Autodesk Inventor part; units mm, degrees
ref_plane "YZ Plane" through (0, 0, 0) normal (1, 0, 0) x (0, 1, 0)
ref_plane "XZ Plane" through (0, 0, 0) normal (0, 1, 0) x (-1, 0, 0)
ref_plane "XY Plane" through (0, 0, 0) normal (0, 0, 1) x (1, 0, 0)
sketch "Sketch1" plane through (0, 0, 0) normal (0, 1, 0) x (-1, 0, 0)
  line L0 (0, 0) -> (-60, 0)
  line L1 (-60, 0) -> (-60, -26)
  line L2 (-60, -26) -> (0, -26)
  line L3 (0, -26) -> (0, 0)
  line L4 (-54, -3.5) -> (-6, -3.5)
  line L5 (-6, -3.5) -> (-6, -22.5)
  line L6 (-6, -22.5) -> (-54, -22.5)
  line L7 (-54, -22.5) -> (-54, -3.5)
  line L8 (-54, -3.5) -> (-6, -22.5) construction
  line L9 (-6, -3.5) -> (-54, -22.5) construction
  point P0 (-30, -13)
  dimension "d0" = 60
  dimension "d2" = 48
  dimension "d3" = 6
  dimension "d4" = 6
  dimension "d36" = 19
  dimension "d37" = 3.5
  dimension "d38" = 3.5
  dimension "d39" = 26
extrude "Extrusion1" add sketch "Sketch1" along normal blind 2 contours L3 L2 L1 L0 | L4 L5 L6 L7
extrude "Extrusion2" add sketch "Sketch1" along normal blind 19
sketch "Sketch2" plane through (0, 2, 0) normal (0, 1, 0) x (1, 0, 0)
  line L0 (6, 3.5) -> (54, 3.5)
  line L1 (54, 22.5) -> (6, 22.5)
  line L2 (54, 3.5) -> (48, 3.5)
  line L3 (48, 3.5) -> (48, 22.5)
  line L4 (48, 22.5) -> (54, 22.5)
  line L5 (54, 22.5) -> (54, 3.5)
  line L6 (6, 3.5) -> (6, 22.5)
  point P0 (0, 0)
  point P1 (48, 3.5)
  dimension "d11" = 42
extrude "Extrusion3" add sketch "Sketch2" along normal blind 3 contours L3 L1 L5 L0
sketch "Sketch3" plane through (0, 0, -3) normal (1, 0, 0) x (0, 0, -1)
  line L0 (-3, 0) -> (23, 0)
  line L1 (23, 0) -> (23, 19)
  line L2 (-3, 19) -> (23, 19)
  line L3 (-3, 0) -> (-3, 19)
  line L4 (2.5, 13) -> (17.5, 13)
  line L5 (17.5, 13) -> (17.5, 5)
  line L6 (17.5, 5) -> (2.5, 5)
  line L7 (2.5, 5) -> (2.5, 13)
  line L8 (2.5, 13) -> (17.5, 5) construction
  line L9 (17.5, 13) -> (2.5, 5) construction
  point P0 (-3, 0)
  point P1 (10, 9)
  point P2 (23, 9.5)
  point P3 (-3, 9.5)
  dimension "d14" = 5
  dimension "d15" = 8
  dimension "d16" = 5.5
  dimension "d17" = 5.5
  dimension "d18" = 15
extrude "Extrusion4" cut sketch "Sketch3" along normal blind 7.5 contours L4 L5 L6 L7
sketch "Sketch4" plane through (60, 0, 0) normal (1, 0, 0) x (0, 0, -1)
  circle A0 centre (7, 12) radius 1.5
  circle A1 centre (19, 12) radius 1.5
  line L0 (0, 0) -> (26, 0)
  line L1 (0, 0) -> (0, 19)
  line L2 (26, 0) -> (26, 19)
  dimension "d21" = 3
  dimension "d22" = 3
  dimension "d25" = 12
  dimension "d26" = 12
  dimension "d27" = 7
  dimension "d28" = 7
extrude "Extrusion5" cut sketch "Sketch4" against normal blind 7.5
fillet "Fillet1" radius 3 4 edges at (0, 9.5, 0) (0, 9.5, -26) (60, 9.5, 0) (60, 9.5, -26)
sketch "Sketch5" plane through (0, 19, 0) normal (0, 1, 0) x (1, 0, 0)
  arc A0 (60, 23) -> (57, 26) centre (57, 23) ccw
  line L0 (57, 26) -> (3, 26)
  arc A1 (3, 26) -> (0, 23) centre (3, 23) ccw
  line L1 (0, 23) -> (0, 3)
  arc A2 (0, 3) -> (3, 0) centre (3, 3) ccw
  line L2 (3, 0) -> (57, 0)
  arc A3 (57, 0) -> (60, 3) centre (57, 3) ccw
  line L3 (60, 3) -> (60, 23)
  line L4 (54, 3.5) -> (6, 3.5)
  line L5 (6, 3.5) -> (6, 22.5)
  line L6 (6, 22.5) -> (54, 22.5)
  line L7 (54, 22.5) -> (54, 3.5)
  circle A4 centre (3, 3) radius 1
  circle A5 centre (3, 23) radius 1
  circle A6 centre (57, 3) radius 1
  circle A7 centre (57, 23) radius 1
  point P0 (0, 0)
  dimension "d30" = 2
  dimension "d31" = 2
  dimension "d32" = 2
  dimension "d33" = 2
extrude "Extrusion6" cut sketch "Sketch5" against normal blind 3 contours A4 | A5 | A6 | A7
sketch "Sketch6" plane through (0, 19, 0) normal (0, 1, 0) x (1, 0, 0)
  circle A0 centre (57, 3) radius 1
  circle A1 centre (3, 23) radius 1
  circle A2 centre (57, 23) radius 1
  circle A3 centre (3, 3) radius 1
  arc A4 (60, 23) -> (57, 26) centre (57, 23) ccw
  line L0 (57, 26) -> (3, 26)
  arc A5 (3, 26) -> (0, 23) centre (3, 23) ccw
  line L1 (0, 23) -> (0, 3)
  arc A6 (0, 3) -> (3, 0) centre (3, 3) ccw
  line L2 (3, 0) -> (57, 0)
  arc A7 (57, 0) -> (60, 3) centre (57, 3) ccw
  line L3 (60, 3) -> (60, 23)
  line L4 (54, 3.5) -> (6, 3.5)
  line L5 (6, 3.5) -> (6, 22.5)
  line L6 (6, 22.5) -> (54, 22.5)
  line L7 (54, 22.5) -> (54, 3.5)
  line L8 (6, 22.5) -> (6, 3.5)
  line L9 (6, 3.5) -> (4.6176, 3.5)
  line L10 (4.6176, 3.5) -> (4.6176, 22.5)
  line L11 (4.6176, 22.5) -> (6, 22.5)
  line L12 (6, 22.5) -> (6, 3.5)
  point P0 (0, 0)
extrude "Extrusion7" cut sketch "Sketch6" against normal blind 17 contours L9 L10 L11 L5
equation "\"d38\" = d37"
equation "\"d26\" = d25"
equation "\"d28\" = d27"
properties part number "bawah"
CAD build for the part. Positions are in the model's coordinates, mm. A direction names the side the tool comes from. Coordinates: 2 decimals unless noted, no trailing zeros. Order: outer loops, then holes, each group sorted by start corner. A loop starts at its lowest first (then second) coordinate and runs counter-clockwise, first axis right, second up. Notation, with made-up numbers: M -2,42.5 L 55,42.5 A15 cw 55,69.5 Z; hole C -22,39 d3. An arc over 180 degrees is marked long. Write each question's results on one line, items separated by ' | '. Start each with the question number.
Q1. Pull direction Z, two halves, no side cores. Call faces 4 (the cylindrical face through (59.1, 9.63, -0.86)), 5 (the flat face through (54, 12, -13)), 6 (the flat face through (30, 9, -26)): +Z half, -Z half, draft (parallel to the pull), parting line (faces both ways), or undercut.
Q2. Drill centre lines: probe 1 along X at (y, z) = (17.25, -23); probe 2 along Z at (x, y) = (3, 18.4); probe 3 along Z at (x, y) = (4, 6.25). Where is each one in solid material? Low to high. Write a range as from..to.
Q3. Cut at C-C (z = -10.75). List the corners of the cut face in (x, y).
Q4. Which spindle directions (+Z, -Z, +X, -X, +Y, -Y) get a long thin tool onto all of the face, cutting with end or side? Do faces 1 (the flat face through (2, 13, -13)), 2 (the flat face through (30, 19, -24)), 3 (the flat face through (3, 16, -23)). Say none if no direction does.
Q5. Cut at B-B (z = -7). List the corners of the cut face in (x, y), then the cut area to 3 significant figures.
Q6. Flat gauge pins, fed straight in: P1, Ø8, axis at x = 43.5, y = 7.5, coming from the +Z side; P2, Ø0.6, axis at x = 57.5, z = -23, coming from the +Y side. Where does each tip first touch, or does it go through?
Q7. Cut at D-D (x = 38). List the corners of the cut face in (y, z).
Q8. Cut at A-A (y = 12). List the corners of the cut face in (x, z).
Found:
1) face 4: +Z half | face 5: undercut | face 6: -Z half
2) probe 1: 0..2, 4..56, 58..60 | probe 2: -26..-24, -22..-4, -2..0 | probe 3: -26..-20.5, -5.5..0
3) outline: M 0,0 L 60,0 L 60,19 L 54,19 L 54,5 L 48,5 L 48,2 L 4.62,2 L 4.62,5 L 0,5 Z; M 0,13 L 4.62,13 L 4.62,19 L 0,19 Z
4) face 1: -X | face 2: +Z, -Z, +X, -X, +Y | face 3: +Y
5) outline: M 0,0 L 60,0 L 60,10.5 L 54,10.5 L 54,5 L 48,5 L 48,2 L 4.62,2 L 4.62,5 L 0,5 Z; M 0,13 L 4.62,13 L 4.62,19 L 0,19 Z; M 54,13.5 L 60,13.5 L 60,19 L 54,19 Z | area: 264 mm²
6) P1: z = 0 | P2: y = 16
7) outline: M 0,-26 L 19,-26 L 19,-22.5 L 2,-22.5 L 2,-3.5 L 19,-3.5 L 19,0 L 0,0 Z
8) outline: M 0,-23 A3 ccw 3,-26 L 57,-26 A3 ccw 60,-23 L 60,-20.5 L 54,-20.5 L 54,-22.5 L 4.62,-22.5 L 4.62,-20.5 L 0,-20.5 Z; M 0,-5.5 L 4.62,-5.5 L 4.62,-3.5 L 54,-3.5 L 54,-5.5 L 60,-5.5 L 60,-3 A3 ccw 57,0 L 3,0 A3 ccw 0,-3 Z; M 54,-17.5 L 60,-17.5 L 60,-8.5 L 54,-8.5 Z
